The model under review builds one solid part; all positions refer to its coordinate system, in mm. A direction names the side the tool comes from. Coordinates: 2 decimals unless noted, no trailing zeros. Order: outer loops, then holes, each group sorted by start corner. A loop starts at its lowest first (then second) coordinate and runs counter-clockwise, first axis right, second up.
from build123d import *

# Parameters (mm, degrees)
F0_W     = 60
F0_H     = 60
F1_DEPTH = 32
F2_R     = 17.5
F3_DEPTH = 64
F4_W     = 20
F4_H     = 20
F5_DEPTH = 60
F6_W     = 35
F6_H     = 10
F7_DEPTH = 60
F8_R     = 10
F9_DEPTH = 96


with BuildPart() as f1:
    # F0 (on Top) → F1 (new body)
    with BuildSketch(Plane.XY):
        Rectangle(F0_W, F0_H)
    extrude(amount=F1_DEPTH)

    # F2 (on face) → F3 (join)
    with BuildSketch(Plane.XY.offset(32)):
        Circle(F2_R)
    extrude(amount=F3_DEPTH)

    # F4 (on face) → F5 (cut)
    with BuildSketch(Plane.XZ.offset(30)):
        with Locations((0, 10)):
            Rectangle(F4_W, F4_H)
    extrude(amount=-F5_DEPTH, mode=Mode.SUBTRACT)

    # F6 (on face) → F7 (cut)
    with BuildSketch(Plane.YZ.offset(30)):
        with Locations((0, 5)):
            Rectangle(F6_W, F6_H)
    extrude(amount=-F7_DEPTH, mode=Mode.SUBTRACT)

    # F8 (on face) → F9 (cut)
    with BuildSketch(Plane.XY.offset(96)):
        Circle(F8_R)
    extrude(amount=-F9_DEPTH, mode=Mode.SUBTRACT)


solid = f1.part
(1) Consider section D-D (y = 4). Give the boundary of the cut face in (x, z), then the cut area to 3 significant figures.
(2) The part is to be moulded in two halves that separate along X. For faces 5 (the face through (-30, 0, 19)), 6 (the face through (-13.887, -10.648, 63.552)), 7 (the face through (-2.17, -9.76, 58.53)), 8 (the face through (-10, 0, 12)), say which applies: +X half, -X half, draft (parallel to the pull), parting line (faces both ways), or undercut.
(3) Insertion check: pin 1 Ø22 at (y, z) = (9.5, 5.5) entering from +X; pin 2 Ø10 at (x, y) = (-0.5, -17.5) entering from -Z; pin 3 Ø4 at (x, y) = (24, 12.5) entering from +Z; pin 4 Ø1 at (y, z) = (-15.5, 46) entering from +X. Each pin has a flat end and moves straight along its axis. Give the tip position at first contact, or say it passes through.
(4) Tool access review of faces 1 (the face through (-14, 14, 32)), 2 (the face through (0, -19, 20)), 3 (the face through (0, 30, 23)), 4 (the face through (-20, 17.5, 5)): name each direction out of +Z, -Z, +X, -X, +Y, -Y from which nothing blocks a thin tool from reaching the whole face with its end or side.
(5) Wall thickness on line 1 (X direction, y = 19, z = 9.5); line 2 (Y direction, x = 0, z = 67); line 3 (Y direction, x = -12, z = 5.5): over which ranges is each line inside the solid? List them lowest first.
(6) Consider section B-B (z = 28). Give the boundary of the cut face in (x, y).
(7) Consider section C-C (z = 15). Give the boundary of the cut face in (x, y).
(8) Consider section A-A (x = 0). Give the boundary of the cut face in (y, z), then the cut area to 3 significant figures.
Findings:
1. outline: (-30, 10) - (-10, 10) - (-10, 20) - (-9.17, 20) - (-9.17, 96) - (-17.04, 96) - (-17.04, 32) - (-30, 32) - close; (9.17, 20) - (10, 20) - (10, 10) - (30, 10) - (30, 32) - (17.04, 32) - (17.04, 96) - (9.17, 96) - close
1. area: 1,910 mm2
2. face 5: -X half
2. face 6: parting line
2. face 7: undercut
2. face 8: undercut
3. pin 1: stops at x = 30
3. pin 2: stops at z = 20
3. pin 3: stops at z = 32
3. pin 4: stops at x = 9.01
4. face 1: +Z
4. face 2: -Z, +Y, -Y
4. face 3: +Z, -Z, +X, -X, +Y
4. face 4: -Z, +X, -X
5. line 1: x = -30 to -10, 10 to 30
5. line 2: y = -17.5 to -10, 10 to 17.5
5. line 3: y = -30 to -17.5, 17.5 to 30
6. outline: (-30, -30) - (30, -30) - (30, 30) - (-30, 30) - close; hole circle Ø20 at (0, 0)
7. outline: (-30, -30) - (-10, -30) - (-10, 30) - (-30, 30) - close; (10, -30) - (30, -30) - (30, 30) - (10, 30) - close
8. outline: (-30, 20) - (-10, 20) - (-10, 96) - (-17.5, 96) - (-17.5, 32) - (-30, 32) - close; (10, 20) - (30, 20) - (30, 32) - (17.5, 32) - (17.5, 96) - (10, 96) - close
8. area: 1,440 mm2
